Geometry: final body of the model. Coordinates: model frame, mm. A direction names the side the tool comes from. Round coordinates to 2 decimals unless told otherwise and drop trailing zeros. Loops run counter-clockwise (first coordinate to the right, second up) from the corner with the lowest first, then second, coordinate; pieces in that order, holes last. Notation, with made-up numbers: (-30.75, 54.5) -> (-16.75, 54.5) arc R13 cw to (-16.75, 65.5) -> close; hole circle Ø1 at (87, 53.25). An arc over 180 degrees is marked (long way). Answer in a Markdown table with one row per item.
```python
from build123d import *

# Parameters (mm, degrees)
SKETCH_R     = 5
PAD_DEPTH    = 12
SKETCH001_R  = 3
POCKET_DEPTH = 10
FILLET_R     = 4
CHAMFER_SIZE = 1
FILLET001_R  = 2


with BuildPart() as part:
    # Sketch → Pad (new body)
    with BuildSketch(Plane.XY):
        Circle(SKETCH_R)
    extrude(amount=PAD_DEPTH)

    # Sketch001 (on Face3 of Pad) → Pocket (cut)
    with BuildSketch(Plane.XY.offset(12)):
        Circle(SKETCH001_R)
    extrude(amount=-POCKET_DEPTH, mode=Mode.SUBTRACT)

    # Fillet
    fillet_edges = [part.edges().sort_by_distance(p)[0] for p in [
        (-5, 0, 0),
    ]]
    fillet(fillet_edges, radius=FILLET_R)

    # Chamfer
    chamfer_edges = [part.edges().sort_by_distance(p)[0] for p in [
        (-5, 0, 12),
    ]]
    chamfer(chamfer_edges, length=CHAMFER_SIZE)

    # Fillet001
    fillet001_edges = [part.edges().sort_by_distance(p)[0] for p in [
        (-3, 0, 2),
    ]]
    fillet(fillet001_edges, radius=FILLET001_R)


solid = part.part
```
Item 1: Pin query (flat end, axial travel): pin 1 Ø6 at (y, z) = (-3.5, 10.5) entering from +X; pin 2 Ø1.5 at (x, z) = (-1.5, 3.5) entering from +Y; pin 3 Ø1.5 at (x, y) = (-1.5, -0.5) entering from +Z. Return the tip coordinate at first contact, or that it passes through.
Answer:
| item | result |
|---|---|
| pin 1 | stops at x = 4.97 |
| pin 2 | stops at y = 4.93 |
| pin 3 | stops at z = 2.51 |
Item 2: Line query: probe 1 along Y at (x, z) = (0, 5.5); probe 2 along X at (y, z) = (2.5, 5.25); probe 3 along X at (y, z) = (2.75, 9.25). Output: solid intervals per line, ascending. Write a range as [from, to].
Answer:
| item | result |
|---|---|
| probe 1 | y = [-5, -3], [3, 5] |
| probe 2 | x = [-4.33, -1.66], [1.66, 4.33] |
| probe 3 | x = [-4.18, -1.2], [1.2, 4.18] |
Item 3: Reachability of faces 1 (the face through (0, 0, 2)), 2 (the face through (0, 0, 0)) from +Z, -Z, +X, -X, +Y, -Y: full face, straight path, thin tool, end or side. Return the list, or none.
Answer:
| item | result |
|---|---|
| face 1 | +Z |
| face 2 | -Z, +X, -X, +Y, -Y |
Item 4: Cut plane A-A (z = 9). Output: boundary loops of the cut face in (x, y), then the cut area to 3 significant figures.
Answer:
| item | result |
|---|---|
| outline | circle Ø10 at (0, 0); hole circle Ø6 at (0, 0) |
| area | 50.3 mm² |
Item 5: Draft query along X for faces 3 (the face through (-1.08, -4.88, 7.45)), 4 (the face through (1, 3, 12)), 5 (the face through (-3, 0, 8)). Return one class per face: pulls with the +X half, pulls with the -X half, needs draft (parallel to the pull), parting line crosses it, or undercut.
Answer:
| item | result |
|---|---|
| face 3 | parting line crosses it |
| face 4 | needs draft |
| face 5 | undercut |
